The listing builds one solid part. Answer for the finished solid, in the listing's coordinates (mm). Give positions to 0.01 mm unless a question says otherwise; leave off trailing zeros. Write each loop counter-clockwise with the first axis right and the second up, starting at its lowest first coordinate (ties: lowest second). Pieces come first, ordered by that corner, then holes. Notation, with made-up numbers: (43, 45.5) - (98, 45.5) arc R14 cw to (98, 51.5) - close; hole circle Ø2 at (42, 39.25). An arc over 180 degrees is marked (long way). Answer in a Markdown table with one row per item. Add a question column.
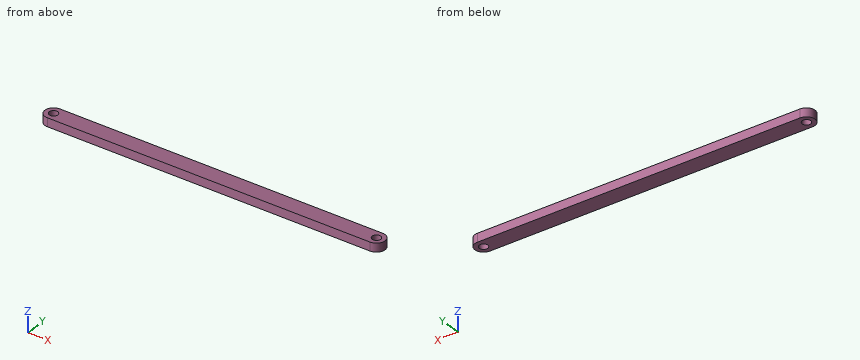
Solid Edge part; units mm, degrees
sketch "Sketch1" plane through (0, 0, 0) normal (0, 0, 1) x (1, 0, 0)
  circle A0 centre (-45.1905, 0) radius 2
  circle A1 centre (106.8795, 0) radius 2
  line L0 (-45.1905, 4) -> (106.8795, 4)
  line L1 (106.8795, -4) -> (-45.1905, -4)
  arc A2 (-45.1905, -4) -> (-45.1905, 4) centre (-45.1905, 0) cw
  arc A3 (106.8795, 4) -> (106.8795, -4) centre (106.8795, 0) cw
extrude "Protrusion1" add sketch "Sketch1" along normal blind 4
1. Straight lines are drawn through the part: L1, parallel to X at y = -0.75, z = 3.6; L2, parallel to X at y = 0.5, z = 2.65; L3, parallel to X at y = 3, z = 3.5. For each, find the intervals that lie inside material, in ascending order. Write a range as [from, to].
2. Section B-B (z = 2) is taken. Give the vertices of the cut face in (x, y).
3. Section A-A (y = 0) is taken. Give the vertices of the cut face in (x, z).
4. Given pin 1 Ø4.5 at (x, y) = (-45.19, 0) entering from -Z, flat-ended and moving along its own axis, determine where the tip first touches the part or whether it passes through.
Geometry check:
| question | item | result |
|---|---|---|
| 1 | L1 | [-49.12, -47.04], [-43.34, 105.03], [108.73, 110.81] |
| 1 | L2 | [-49.16, -47.13], [-43.25, 104.94], [108.82, 110.85] |
| 1 | L3 | [-47.84, 109.53] |
| 2 | outline | (-45.19, -4) - (106.88, -4) arc R4 ccw to (106.88, 4) - (-45.19, 4) arc R4 ccw to start; hole circle Ø4 at (-45.19, 0); hole circle Ø4 at (106.88, 0) |
| 3 | outline | (-49.19, 0) - (-47.19, 0) - (-47.19, 4) - (-49.19, 4) - close; (-43.19, 0) - (104.88, 0) - (104.88, 4) - (-43.19, 4) - close; (108.88, 0) - (110.88, 0) - (110.88, 4) - (108.88, 4) - close |
| 4 | pin 1 | z = 0 |
